Model file for the job. Use its own axes, mm. Face numbers are marked on the shaded views. A direction names the side the tool comes from. Round coordinates to 2 decimals unless told otherwise and drop trailing zeros. One line per item, written item: value.
from build123d import *

# Parameters (mm, degrees)
SKETCH1_R                = 22.7203
BOSS_EXTRUDE2_DEPTH      = 4.7625
FILLET1_R                = 3.175
SKETCH2_W                = 14.732
SKETCH2_H                = 10.414
CUT_EXTRUDE2_DEPTH       = 12.7
CIRPATTERN1_COUNT        = 5
SKETCH4_R                = 1.143
CUT_EXTRUDE4_DEPTH       = 9.525
CIRPATTERN2_COUNT        = 5
SKETCH5_R                = 3.9751
CUT_EXTRUDE5_DEPTH       = 33.480350535
SKETCH6_R                = 2.159
CUT_EXTRUDE7_DEPTH       = 33.480350535
BOSS_EXTRUDE4_REACH      = 39.999
FILLET2_R                = 0.127
CIRPATTERN5_COUNT        = 5
FILLET2_OF_CIRPATTERN5_R = 0.127
CUT_EXTRUDE8_DEPTH       = 2.54


with BuildPart() as part:
    # Sketch1 → Boss-Extrude2 (new body)
    with BuildSketch(Plane.XY):
        Circle(SKETCH1_R)
    extrude(amount=-BOSS_EXTRUDE2_DEPTH)

    # Fillet1
    fillet1_edges = [part.edges().sort_by_distance(p)[0] for p in [
        (-22.7203, 0, -4.7625),
    ]]
    fillet(fillet1_edges, radius=FILLET1_R)

    # Sketch2 → Cut-Extrude2 (cut)
    with BuildSketch(Plane.XY):
        with Locations((0, 18.7833)):
            Rectangle(SKETCH2_W, SKETCH2_H)
    cut_extrude2 = extrude(amount=-CUT_EXTRUDE2_DEPTH, mode=Mode.SUBTRACT)

    # CirPattern1: Cut-Extrude2 ×5 about axis
    cirpattern1_axis = Axis((0, 0, 0), (0, 0, 1))
    for i in range(1, CIRPATTERN1_COUNT):
        add(cut_extrude2.rotate(cirpattern1_axis, i * 360 / CIRPATTERN1_COUNT), mode=Mode.SUBTRACT)

    # Sketch4 → Cut-Extrude4 (cut, symmetric)
    with BuildSketch(Plane(origin=(0, 0, 0), x_dir=(0, 0, -1), z_dir=(1, 0, 0))):
        with Locations((0, 19.4183)):
            Circle(SKETCH4_R)
    cut_extrude4 = extrude(amount=CUT_EXTRUDE4_DEPTH, both=True, mode=Mode.SUBTRACT)

    # CirPattern2: Cut-Extrude4 ×5 about axis
    cirpattern2_axis = Axis((0, 0, 0), (0, 0, 1))
    for i in range(1, CIRPATTERN2_COUNT):
        add(cut_extrude4.rotate(cirpattern2_axis, i * 360 / CIRPATTERN2_COUNT), mode=Mode.SUBTRACT)

    # Sketch5 → Cut-Extrude5 (cut, through all)
    with BuildSketch(Plane.XY):
        Circle(SKETCH5_R)
    extrude(amount=-CUT_EXTRUDE5_DEPTH, mode=Mode.SUBTRACT)

    # Sketch6 → Cut-Extrude7 (cut, through all)
    with BuildSketch(Plane(origin=(0, 0, -4.7625), x_dir=(-1, 0, 0), z_dir=(0, 0, -1))):
        with Locations((0, -9.525)):
            Circle(SKETCH6_R)
        with Locations((-8.248891971, 4.7625)):
            Circle(SKETCH6_R)
        with Locations((8.248891971, 4.7625)):
            Circle(SKETCH6_R)
    extrude(amount=-CUT_EXTRUDE7_DEPTH, mode=Mode.SUBTRACT)

    # Sketch10 → Boss-Extrude4 (add, up to next)
    with BuildSketch(Plane.ZY.offset(-7.366), mode=Mode.PRIVATE) as boss_extrude4_sk1:
        with BuildLine():
            Line((-4.7625, 13.5763), (0, 13.5763))
            Line((0, 13.5763), (0, 13.7033))
            ThreePointArc((0, 13.7033), (-2.7025038, 14.38265722), (-4.7625, 16.259214887))
            Line((-4.7625, 16.259214887), (-4.7625, 13.5763))
        make_face()
    boss_extrude4_tool1 = extrude(boss_extrude4_sk1.sketch, amount=BOSS_EXTRUDE4_REACH, mode=Mode.PRIVATE) - part.part
    boss_extrude4 = boss_extrude4_tool1.solids().sort_by_distance((7.366, 14.314807, -3.452063))[0]
    add(boss_extrude4)

    # Fillet2
    fillet2_edges = [part.edges().sort_by_distance(p)[0] for p in [
        (0, 16.259214887, -4.7625),
    ]]
    fillet(fillet2_edges, radius=FILLET2_R)

    # CirPattern5: Boss-Extrude4 ×5 about axis
    cirpattern5_axis = Axis((0, 0, 0), (0, 0, 1))
    for i in range(1, CIRPATTERN5_COUNT):
        add(boss_extrude4.rotate(cirpattern5_axis, i * 360 / CIRPATTERN5_COUNT))

    # Fillet2 of CirPattern5
    fillet2_of_cirpattern5_edges = [part.edges().sort_by_distance(p)[0] for p in [
        (-15.463432268, 5.024373715, -4.7625),
        (-9.556926725, -13.153981159, -4.7625),
        (9.556926725, -13.153981159, -4.7625),
        (15.463432268, 5.024373715, -4.7625),
    ]]
    fillet(fillet2_of_cirpattern5_edges, radius=FILLET2_OF_CIRPATTERN5_R)

    # Sketch7 → Cut-Extrude8 (cut)
    with BuildSketch(Plane(origin=(0, 0, -4.7625), x_dir=(-1, 0, 0), z_dir=(0, 0, -1))):
        Polygon((-10.815213918, 0.3175), (-5.682570024, 0.3175), (-3.116248078, 4.7625), (-5.682570024, 9.2075), (-10.815213918, 9.2075), (-13.381535864, 4.7625), align=None)
        Polygon((5.132643893, -9.525), (2.566321947, -5.08), (-2.566321947, -5.08), (-5.132643893, -9.525), (-2.566321947, -13.97), (2.566321947, -13.97), align=None)
        Polygon((5.682570024, 9.2075), (3.116248078, 4.7625), (5.682570024, 0.3175), (10.815213918, 0.3175), (13.381535864, 4.7625), (10.815213918, 9.2075), align=None)
    extrude(amount=-CUT_EXTRUDE8_DEPTH, mode=Mode.SUBTRACT)


solid = part.part
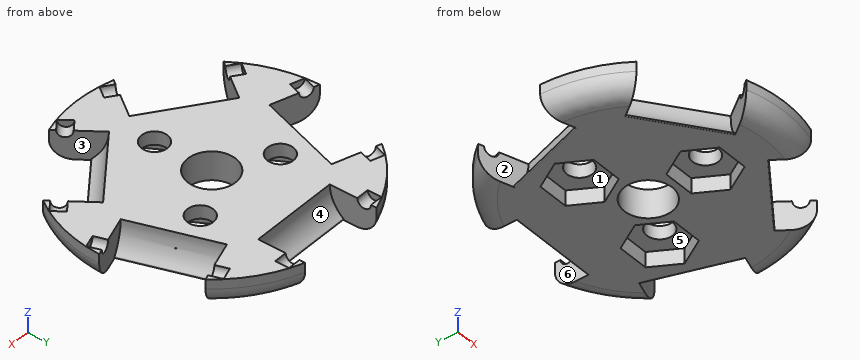
1. Wall check: probe 1 along Y at (x, z) = (-1, -1.3); probe 2 along Y at (x, z) = (0, -2.5); probe 3 along X at (y, z) = (5, -3.05). Give the ranges that are in metal, low to high. Write a range as [from, to].
Report:
probe 1: [-22.7, -11.44], [-7.61, -3.85], [3.85, 13.85]
probe 2: [-22.59, -13.97], [-5.08, -3.98], [3.98, 14.28]
probe 3: [-13.71, -13.24], [-3.25, 3.25], [13.24, 13.71]
2. Drop flat-ended pins along their axis: pin 1 (4.5 mm diameter, centred on x = -1.5, y = -11, fed in from -Z); pin 2 (2 mm diameter, centred on y = 6.5, z = -2, fed in from -X); pin 3 (2.5 mm diameter, centred on x = 0, y = -9.525, fed in from -Z); pin 4 (1.3 mm diameter, centred on x = -1, z = -3, fed in from -Y). Give the stop position or say it passes through.
Report:
pin 1: z = -2.22
pin 2: x = -13.27
pin 3: through
pin 4: y = -22.61
3. Band-saw the part on A-A on x = 0. State how many separate pieces and enclosed holes the cut face has, plus the area to 3 significant figures.
Report:
separate pieces: 3
enclosed holes: 0
area: 105 mm²
4. Mould opens along Y. For the marked faces 4, 5 and 6 say: released by +Y, released by -Y, zero draft, split by the parting line, or undercut.
Report:
face 4: released by +Y
face 5: undercut
face 6: zero draft
5. Tool access for the marked faces 1, 2 and 3: list every direction of +Z, -Z, +X, -X, +Y, -Y with a clear straight run to the whole face (end or side of a thin tool).
Report:
face 1: -Z
face 2: +Z, -X
face 3: +Z, +X
